Study the drawing (mm; zero at the part's minimum x, y, z) and answer. Give positions to 0.01 mm unless a question says otherwise; leave off trailing zeros. Order: outer loops, then holes, each group sorted by start corner. A loop starts at its lowest first (then second) coordinate and runs counter-clockwise, first axis right, second up. Notation, with made-up numbers: (78, -19.75) -> (101, -19.75) arc R29 cw to (101, 12.25) -> close; hole circle Ø6 at (47, -24.5). An arc over 180 degrees is marked (long way). Answer as CSV lines item,"result". Start each with the question number.
1. A cutting plane is placed at C-C (y = 30). Give the vertices of the cut face in (x, z).
2. A cutting plane is placed at B-B (z = 10.25). Give the vertices of the cut face in (x, y).
3. For a pull along X with two mould halves and no side action, classify the marked faces 1, 2 and 3 as released by +X, released by -X, zero draft, split by the parting line, or undercut.
4. A cutting plane is placed at A-A (x = 35.5). Give the vertices of the cut face in (y, z).
5. Flat-ended cylindrical pins translate along their axes: pin 1 (2 mm diameter, centred on y = 8, z = 12, fed in from +X); pin 2 (1.3 mm diameter, centred on x = 15.5, y = 1, fed in from +Z); pin 3 (8 mm diameter, centred on x = 20.5, z = 6.5, fed in from -Y). Find the tip coordinate at first contact, or state that the pin passes through.
6. A cutting plane is placed at D-D (x = 42). Give the vertices of the cut face in (y, z).
7. Find the intervals of material crossed by L1, parallel to Y at x = 21, z = 8; L2, parallel to Z at x = 17.5, y = 2 (1 decimal); L3, parallel to Z at x = 7, y = 24 (1 decimal), in increasing order.
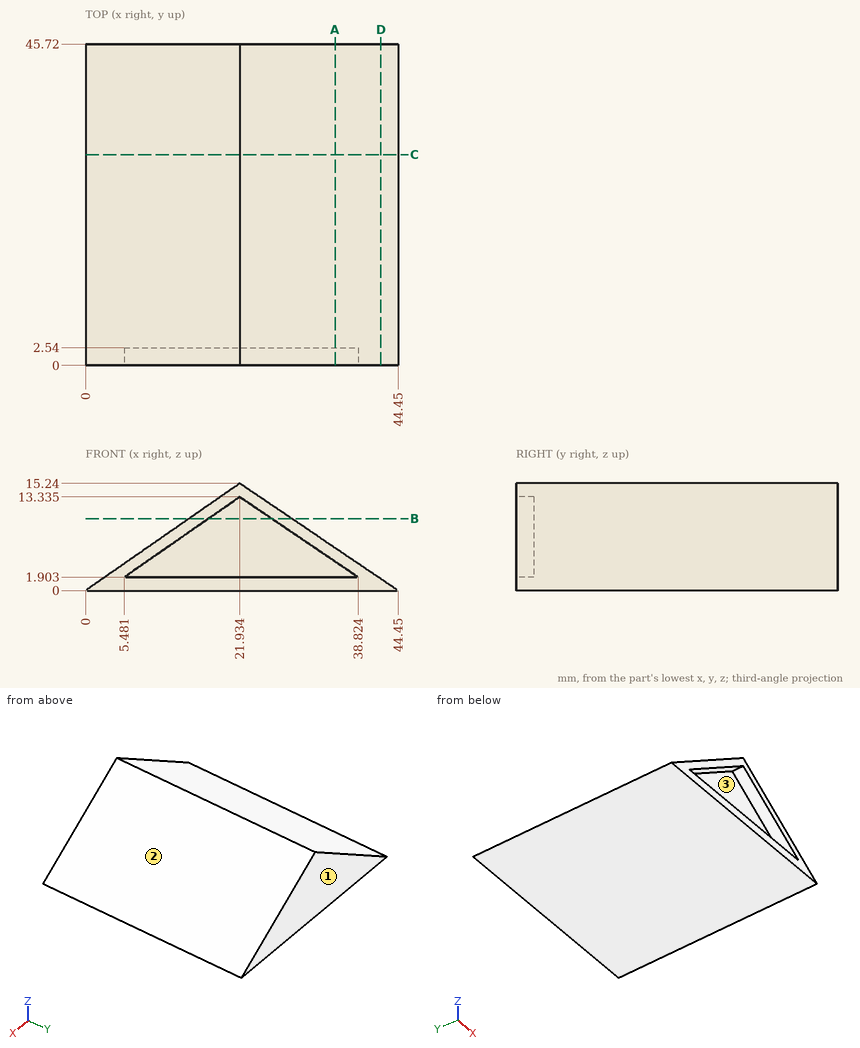
Answer sheet:
1,outline,"(0, 0) -> (44.45, 0) -> (21.93, 15.24) -> close"
2,outline,"(14.75, 0) -> (17.49, 0) -> (17.49, 2.54) -> (26.49, 2.54) -> (26.49, 0) -> (29.31, 0) -> (29.31, 45.72) -> (14.75, 45.72) -> close"
3,face 1,"zero draft"
3,face 2,"released by +X"
3,face 3,"undercut"
4,outline,"(0, 0) -> (45.72, 0) -> (45.72, 6.06) -> (0, 6.06) -> (0, 4.15) -> (2.54, 4.15) -> (2.54, 1.9) -> (0, 1.9) -> close"
5,pin 1,"stops at x = 28.2"
5,pin 2,"stops at z = 11.22"
5,pin 3,"stops at y = 2.54"
6,outline,"(0, 0) -> (45.72, 0) -> (45.72, 1.66) -> (0, 1.66) -> close"
7,L1,"y = 2.54 to 45.72"
7,L2,"z = 0 to 1.9, 10.3 to 12.2"
7,L3,"z = 0 to 4.9"
